```python
from build123d import *

# Parameters (mm, degrees)
SKETCH1_R           = 1.13211215
BOSS_EXTRUDE1_DEPTH = 5.9944


with BuildPart() as part:
    # Sketch1 → Boss-Extrude1 (new body)
    with BuildSketch(Plane.XY):
        Polygon((68.439590063, -10.224157235), (68.439590063, 68.128182765), (-8.002589937, 67.93922998), (-8.002589937, -10.41311002), align=None)
        with Locations((-5.444904937, -5.83350772)):
            Circle(SKETCH1_R, mode=Mode.SUBTRACT)
        with Locations((-5.444904937, 6.28184228)):
            Circle(SKETCH1_R, mode=Mode.SUBTRACT)
        with Locations((12.862735063, 6.28184228)):
            Circle(SKETCH1_R, mode=Mode.SUBTRACT)
        with Locations((12.862735063, -5.83350772)):
            Circle(SKETCH1_R, mode=Mode.SUBTRACT)
        with Locations((47.574265063, -5.649939535)):
            Circle(SKETCH1_R, mode=Mode.SUBTRACT)
        with Locations((47.574265063, 6.465410465)):
            Circle(SKETCH1_R, mode=Mode.SUBTRACT)
        with Locations((65.881905063, 6.465410465)):
            Circle(SKETCH1_R, mode=Mode.SUBTRACT)
        with Locations((65.881905063, -5.649939535)):
            Circle(SKETCH1_R, mode=Mode.SUBTRACT)
        with Locations((47.574265063, 51.433230465)):
            Circle(SKETCH1_R, mode=Mode.SUBTRACT)
        with Locations((47.574265063, 63.548580465)):
            Circle(SKETCH1_R, mode=Mode.SUBTRACT)
        with Locations((65.881905063, 63.548580465)):
            Circle(SKETCH1_R, mode=Mode.SUBTRACT)
        with Locations((65.881905063, 51.433230465)):
            Circle(SKETCH1_R, mode=Mode.SUBTRACT)
        with Locations((12.862735063, 51.24966228)):
            Circle(SKETCH1_R, mode=Mode.SUBTRACT)
        with Locations((12.862735063, 63.36501228)):
            Circle(SKETCH1_R, mode=Mode.SUBTRACT)
        with Locations((-5.444904937, 63.36501228)):
            Circle(SKETCH1_R, mode=Mode.SUBTRACT)
        with Locations((-5.444904937, 51.24966228)):
            Circle(SKETCH1_R, mode=Mode.SUBTRACT)
    extrude(amount=BOSS_EXTRUDE1_DEPTH)


solid = part.part
```
Could you check a few things on this model? Use its own coordinates, in mm. Coordinates: 2 decimals unless noted, no trailing zeros. Write item = value, one per line. Start each with the question number.
(1) Will these pins go through, and if not, where does the flat tip stop? pin 1 (2.5 mm diameter, centred on x = -5.44, y = 6.28, fed in from +Z); pin 2 (2 mm diameter, centred on x = 12.86, y = 63.37, fed in from -Z).
(2) We'd pull the mould along X, two halves only. Please class faces 1 (the face through (30, 29, 0)), 2 (the face through (-8.003, 29, 3)), 3 (the face through (47.329, 62.443, 2.955)), 4 (the face through (68.44, 28, 3)): released by +X, released by -X, zero draft, split by the parting line, or undercut.
(3) I need wall thicknesses on line 1 (Y direction, x = 48.5, z = 0.95); line 2 (Y direction, x = 59.5, z = 5.1); line 3 (Y direction, x = -4.5, z = 3.1). Which ranges of each line are inside material? Lowest first, please. Write a range as [from, to].
Result set:
q1.pin_1 = 5.99
q1.pin_2 = through
q2.face_1 = zero draft
q2.face_2 = released by -X
q2.face_3 = undercut
q2.face_4 = released by +X
q3.line_1 = [-10.27, -6.3], [-5, 5.81], [7.12, 50.78], [52.08, 62.9], [64.2, 68.08]
q3.line_2 = [-10.25, 68.11]
q3.line_3 = [-10.4, -6.46], [-5.21, 5.66], [6.91, 50.63], [51.87, 62.74], [63.99, 67.95]
